Part model, mm, in its own coordinate system. Face numbers are marked on the shaded views. A direction names the side the tool comes from. Coordinates: 2 decimals unless noted, no trailing zeros. Loops run counter-clockwise (first coordinate to the right, second up) from the corner with the lowest first, then second, coordinate; pieces in that order, holes last. Notation, with made-up numbers: M -35.5,5.25 L -11.5,5.25 A23 cw -11.5,32.25 Z; hole C -37.5,15.5 d4. An arc over 180 degrees is marked long. Use CSV: the item, a comma, the result in double quotes. Start each with the question number.
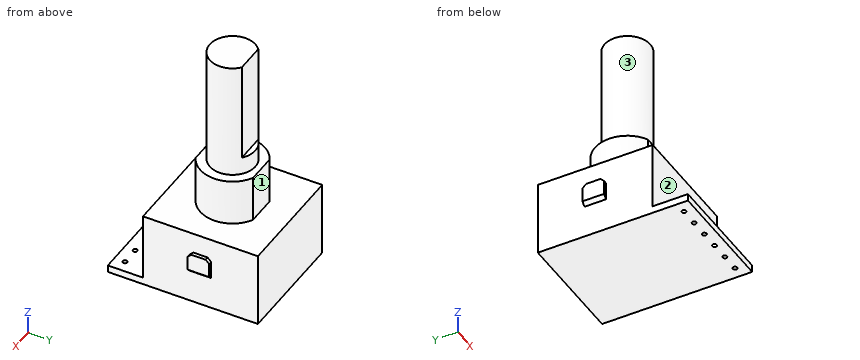
from build123d import *

# Parameters (mm, degrees)
F0_W      = 16
F0_H      = 20.9
F1_DEPTH  = 1
F2_W      = 16
F2_H      = 16
F3_DEPTH  = 9.5
F5_DEPTH  = 6.5
F6_R      = 3.175
F7_DEPTH  = 16.5
F9_DEPTH  = 14
F10_R     = 0.3
F11_DEPTH = 1
F12_W     = 3
F12_H     = 3
F13_DEPTH = 0.5
F14_W     = 3
F14_H     = 3
F15_DEPTH = 0.5
F16_SIZE  = 0.5
F17_SIZE  = 0.49999
F18_SIZE  = 0.49999
F19_SIZE  = 0.5


# Not quite as in the source:
# - a fillet or chamfer is up to 0.001 mm smaller than in the source, because OpenCascade refuses the exact size


with BuildPart() as f1:
    # F0 (on Top) → F1 (new body)
    with BuildSketch(Plane.XY):
        with Locations((0, -2.45)):
            Rectangle(F0_W, F0_H)
    extrude(amount=F1_DEPTH)

    # F2 (on face) → F3 (join)
    with BuildSketch(Plane.XY.offset(1)):
        Rectangle(F2_W, F2_H)
    extrude(amount=F3_DEPTH)

    # F4 (on face) → F5 (join)
    with BuildSketch(Plane.XY.offset(10.5)):
        with BuildLine():
            Line((2.0615528128, 4), (-2.0615528128, 4))
            ThreePointArc((-2.0615528128, 4), (-4.5, 0), (-2.0615528128, -4))
            Line((-2.0615528128, -4), (2.0615528128, -4))
            ThreePointArc((2.0615528128, -4), (4.5, 0), (2.0615528128, 4))
        make_face()
    extrude(amount=F5_DEPTH)

    # F6 (on face) → F7 (join)
    with BuildSketch(Plane.XY.offset(17)):
        Circle(F6_R)
    extrude(amount=F7_DEPTH)

    # F8 (on face) → F9 (cut)
    with BuildSketch(Plane.XY.offset(33.5)):
        with BuildLine():
            ThreePointArc((2.0493901532, 2.425), (0, 3.175), (-2.0493901532, 2.425))
            Line((-2.0493901532, 2.425), (2.0493901532, 2.425))
        make_face()
    extrude(amount=-F9_DEPTH, mode=Mode.SUBTRACT)

    # F10 (on face) → F11 (cut, through all)
    with BuildSketch(Plane(origin=(0, 0, 0), x_dir=(1, 0, 0), z_dir=(0, 0, -1))):
        with Locations((-6.35, 11.43)):
            Circle(F10_R)
        with Locations((-3.81, 11.43)):
            Circle(F10_R)
        with Locations((-1.27, 11.43)):
            Circle(F10_R)
        with Locations((1.27, 11.43)):
            Circle(F10_R)
        with Locations((3.81, 11.43)):
            Circle(F10_R)
        with Locations((6.35, 11.43)):
            Circle(F10_R)
    extrude(amount=-F11_DEPTH, mode=Mode.SUBTRACT)

    # F12 (on face) → F13 (join)
    with BuildSketch(Plane(origin=(-8, 0, 0), x_dir=(0, -1, 0), z_dir=(-1, 0, 0))):
        with Locations((0, 6.1)):
            Rectangle(F12_W, F12_H)
    extrude(amount=F13_DEPTH)

    # F14 (on face) → F15 (join)
    with BuildSketch(Plane.YZ.offset(8)):
        with Locations((0, 6.1)):
            Rectangle(F14_W, F14_H)
    extrude(amount=F15_DEPTH)

    # F16
    f16_edges = [f1.edges().sort_by_distance(p)[0] for p in [
        (-8.25, 1.5, 7.6),
        (-8.25, -1.5, 7.6),
    ]]
    chamfer(f16_edges, length=F16_SIZE)

    # F17 (size 0.5 in the source; OpenCascade refuses exactly that, so slightly less here)
    f17_edges = [f1.edges().sort_by_distance(p)[0] for p in [
        (-8.5, 0, 4.6),
    ]]
    chamfer(f17_edges, length=F17_SIZE)

    # F18 (size 0.5 in the source; OpenCascade refuses exactly that, so slightly less here)
    f18_edges = [f1.edges().sort_by_distance(p)[0] for p in [
        (8.5, 0, 4.6),
    ]]
    chamfer(f18_edges, length=F18_SIZE)

    # F19
    f19_edges = [f1.edges().sort_by_distance(p)[0] for p in [
        (8.25, 1.5, 7.6),
        (8.25, -1.5, 7.6),
    ]]
    chamfer(f19_edges, length=F19_SIZE)


solid = f1.part
1. Slice it at D-D, the plane x = -7.5. List the corners of the cut face in (y, z), and give its area (3 significant figures).
2. Tool access for the marked faces 1, 2 and 3: list every direction of +Z, -Z, +X, -X, +Y, -Y with a clear straight run to the whole face (end or side of a thin tool).
3. Wall check: probe 1 along Y at (x, z) = (-3.81, 0.7); probe 2 along Z at (x, y) = (-6.75, -3); probe 3 along Z at (x, y) = (3.75, -0.5). Give the ranges that are in metal, low to high.
4. Slice it at C-C, the plane z = 5.5. List the corners of the cut face in (x, y).
5. Pin check, flat tips, straight feed: pin 1 (12 mm diameter, centred on y = 3, z = 5, fed in from +X); pin 2 (5 mm diameter, centred on x = 0.5, z = 5.5, fed in from -Y); pin 3 (5 mm diameter, centred on y = -6, z = 5, fed in from +X); pin 4 (2 mm diameter, centred on x = 0.5, z = 15, fed in from -Y). Stop position of each tip, or through.
6. Slice it at A-A, the plane x = 0. List the corners of the cut face in (y, z) (3 decimals), and give its area (3 significant figures).
Found:
1,outline,"M -12.9,0 L 8,0 L 8,10.5 L -8,10.5 L -8,1 L -12.9,1 Z"
1,area,"173 mm^2"
2,face 1,"+Z, +X, -X, +Y"
2,face 2,"+Z, +X, -X, -Y"
2,face 3,"+Z"
3,probe 1,"-12.9 to -11.73, -11.13 to 8"
3,probe 2,"0 to 10.5"
3,probe 3,"0 to 17"
4,outline,"M -8.5,-1.5 L -8,-1.5 L -8,-8 L 8,-8 L 8,-1.5 L 8.5,-1.5 L 8.5,1.5 L 8,1.5 L 8,8 L -8,8 L -8,1.5 L -8.5,1.5 Z"
5,pin 1,"x = 8.5"
5,pin 2,"y = -8"
5,pin 3,"x = 8"
5,pin 4,"y = -4"
6,outline,"M -12.9,0 L 8,0 L 8,10.5 L 4,10.5 L 4,17 L 3.175,17 L 3.175,19.5 L 2.425,19.5 L 2.425,33.5 L -3.175,33.5 L -3.175,17 L -4,17 L -4,10.5 L -8,10.5 L -8,1 L -12.9,1 Z"
6,area,"319 mm^2"
